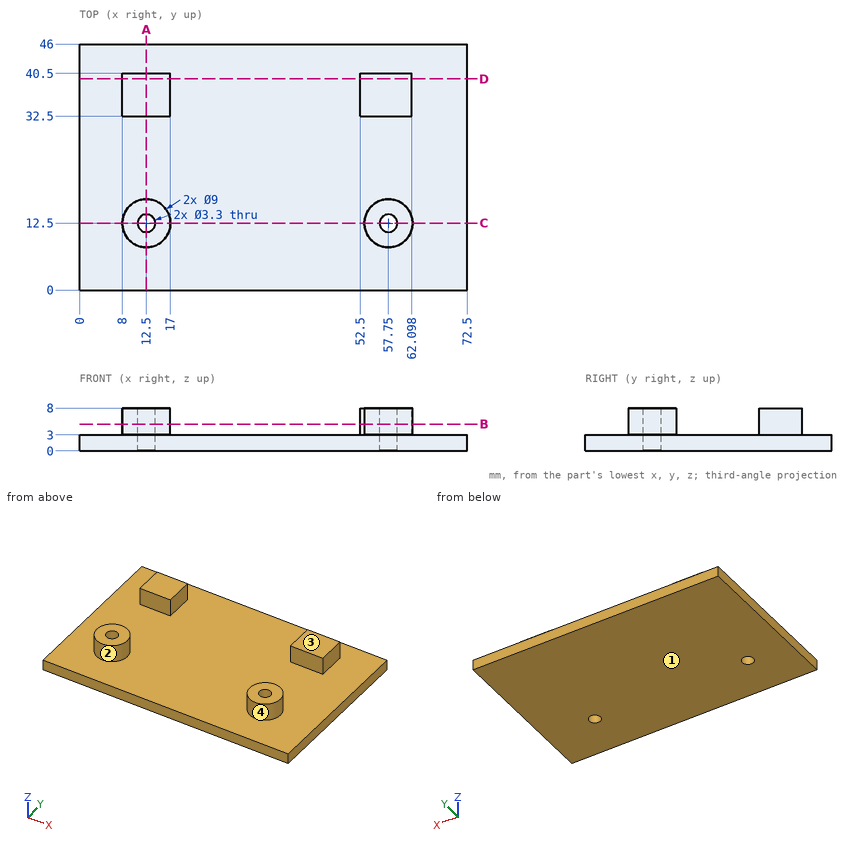
The figure shows three views and two pictorial views of one solid part (mm, origin at its lowest corner). Answer the questions. A direction names the side the tool comes from. Round coordinates to 2 decimals unless told otherwise and drop trailing zeros. Loops run counter-clockwise (first coordinate to the right, second up) from the corner with the lowest first, then second, coordinate; pieces in that order, holes last. Notation, with made-up numbers: M 34,45.5 L 64,45.5 A14 cw 64,60.5 Z; hole C 33,-5 d3. An arc over 180 degrees is marked long. Return JSON: item names as keys, results as strings.
Q1. Find the intervals of material crossed by line 1 along Y through (x, z) = (12.5, 3.5); line 2 along X through (y, z) = (12.5, 1.75); line 3 along X through (y, z) = (12.5, 3.75), in increasing order. Write a range as from..to.
Results list:
{"line 1": "y = 8..10.85, 14.15..17, 32.5..40.5", "line 2": "x = 0..10.85, 14.15..56.1, 59.4..72.5", "line 3": "x = 8..10.85, 14.15..17, 53.25..56.1, 59.4..62.25"}
Q2. Find section D-D, the plane y = 39.5. Determine the outline of the cut face in (x, z).
Results list:
{"outline": "M 0,0 L 72.5,0 L 72.5,3 L 62.1,3 L 62.1,8 L 52.5,8 L 52.5,3 L 17,3 L 17,8 L 8,8 L 8,3 L 0,3 Z"}
Q3. Which of the six approach directions +Z, -Z, +X, -X, +Y, -Y give full straight-line access (tool end or side, diameter ignored) to the marked faces 3 and 4?
Results list:
{"face 3": "+Z, +X, -X, +Y, -Y", "face 4": "+Z"}
Q4. Find section A-A, the plane x = 12.5. Determine the outline of the cut face in (y, z).
Results list:
{"outline": "M 0,0 L 10.85,0 L 10.85,8 L 8,8 L 8,3 L 0,3 Z; M 14.15,0 L 46,0 L 46,3 L 40.5,3 L 40.5,8 L 32.5,8 L 32.5,3 L 17,3 L 17,8 L 14.15,8 Z"}
Q5. The mould has two halves that part along X. Classify the marked faces 1 and 2: released by +X, released by -X, zero draft, split by the parting line, or undercut.
Results list:
{"face 1": "zero draft", "face 2": "undercut"}
Q6. Find section B-B, the plane z = 5. Determine the outline of the cut face in (x, y), plus the area to 3 significant figures.
Results list:
{"outline": "C 12.5,12.5 d9; M 8,32.5 L 17,32.5 L 17,40.5 L 8,40.5 Z; M 52.5,32.5 L 62.1,32.5 L 62.1,40.5 L 52.5,40.5 Z; C 57.75,12.5 d9; hole C 12.5,12.5 d3.3; hole C 57.75,12.5 d3.3", "area": "259 mm2"}
Q7. Find section C-C, the plane y = 12.5. Determine the outline of the cut face in (x, z), plus the area to 3 significant figures.
Results list:
{"outline": "M 0,0 L 10.85,0 L 10.85,8 L 8,8 L 8,3 L 0,3 Z; M 14.15,0 L 56.1,0 L 56.1,8 L 53.25,8 L 53.25,3 L 17,3 L 17,8 L 14.15,8 Z; M 59.4,0 L 72.5,0 L 72.5,3 L 62.25,3 L 62.25,8 L 59.4,8 Z", "area": "255 mm2"}
Q8. Each of these flat-tipped pins is pushed along its axis until it touches: pin 1 Ø2.5 at (y, z) = (37.5, 5.5) entering from -X; pin 2 Ø4 at (x, y) = (21, 37) entering from +Z; pin 3 Ø4 at (y, z) = (35, 6.5) entering from +X; pin 4 Ø2.5 at (x, y) = (57.75, 12.5) entering from -Z. Where does it stop, or does it pass through?
Results list:
{"pin 1": "stops at x = 8", "pin 2": "stops at z = 3", "pin 3": "stops at x = 62.1", "pin 4": "passes through"}
